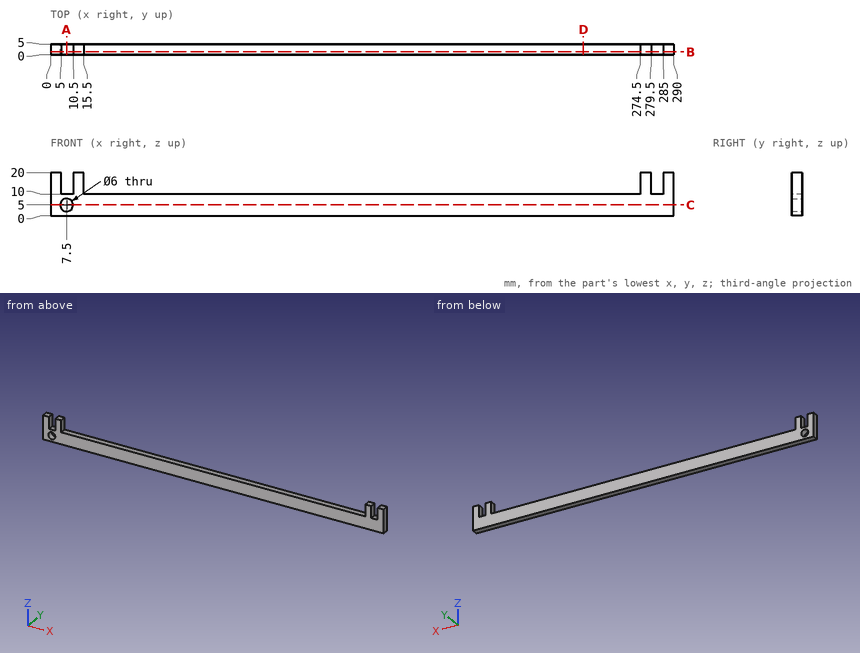
Part print with two shaded views. Sizes in mm from the minimum x, y, z corner. Round coordinates to 2 decimals unless told otherwise and drop trailing zeros. Order: outer loops, then holes, each group sorted by start corner. A loop starts at its lowest first (then second) coordinate and runs counter-clockwise, first axis right, second up. Notation, with made-up numbers: M 23,5.5 L 75,5.5 A29 ccw 75,33.5 Z; hole C 20.25,-38 d1. An arc over 180 degrees is marked long. Put each result on its own line as item: value. Start each with the question number.
1. Slice it at C-C on z = 5. List the corners of the cut face in (x, y), then the cut area to 3 significant figures.
2. Slice it at B-B on y = 1.3. List the corners of the cut face in (x, z).
3. Drop flat-ended pins along their axis: pin 1 (1.5 mm diameter, centred on x = 6.5, y = 2, fed in from +Z); pin 2 (9.5 mm diameter, centred on x = 7.5, z = 5, fed in from -Y). Give the stop position or say it passes through.
4. Slice it at D-D on x = 248. List the corners of the cut face in (y, z).
5. Slice it at A-A on x = 7.5. List the corners of the cut face in (y, z), then the cut area to 3 significant figures.
6. Drill centre lines: probe 1 along X at (y, z) = (3.05, 11.75); probe 2 along Z at (x, y) = (7.5, 3.3); probe 3 along Z at (x, y) = (245.5, 0.6). Where is each one in solid material? Low to high. Write a range as [from, to].
Findings:
1. outline: M 0,0 L 4.5,0 L 4.5,5 L 0,5 Z; M 10.5,0 L 290,0 L 290,5 L 10.5,5 Z
1. area: 1,420 mm2
2. outline: M 0,0 L 290,0 L 290,20 L 285,20 L 285,10 L 279.5,10 L 279.5,20 L 274.5,20 L 274.5,10 L 15.5,10 L 15.5,20 L 10.5,20 L 10.5,10 L 5,10 L 5,20 L 0,20 Z; hole C 7.5,5 d6
3. pin 1: z = 10
3. pin 2: y = 0
4. outline: M 0,0 L 5,0 L 5,10 L 0,10 Z
5. outline: M 0,0 L 5,0 L 5,2 L 0,2 Z; M 0,8 L 5,8 L 5,10 L 0,10 Z
5. area: 20.0 mm2
6. probe 1: [0, 5], [10.5, 15.5], [274.5, 279.5], [285, 290]
6. probe 2: [0, 2], [8, 10]
6. probe 3: [0, 10]
